```python
from build123d import *

# Parameters (mm, degrees)
F0_W     = 200
F0_H     = 172
F0_R     = 7.5
F1_DEPTH = 15
F2_T     = 2.5
F3_R     = 5


# Not quite as in the source:
# - a shell that OpenCascade refuses in one call is made with other operations: the cavity is built on its own and cut out


with BuildPart() as f1:
    # F0 (on Top) → F1 (new body)
    with BuildSketch(Plane.XY):
        with Locations((100, 86)):
            Rectangle(F0_W, F0_H)
        with Locations((11, 11)):
            Circle(F0_R, mode=Mode.SUBTRACT)
        with Locations((189, 11)):
            Circle(F0_R, mode=Mode.SUBTRACT)
        with Locations((11, 161)):
            Circle(F0_R, mode=Mode.SUBTRACT)
        with Locations((189, 161)):
            Circle(F0_R, mode=Mode.SUBTRACT)
    extrude(amount=F1_DEPTH)

    # F2: shell of thickness 2.5, made by hand


with BuildPart() as f2_core1:
    # F2_t2: copy of F1
    add(f1.part)

    # the walls: a layer under each face that stays
    f2_faces = [f2_core1.faces().sort_by_distance(p)[0] for p in [
        (0, 86, 7.5),
        (100, 0, 7.5),
        (200, 86, 7.5),
        (100, 172, 7.5),
        (3.5, 11, 7.5),
        (181.5, 11, 7.5),
        (3.5, 161, 7.5),
        (181.5, 161, 7.5),
        (100, 86, 0),
    ]]
    thicken(f2_faces, amount=-F2_T, mode=Mode.SUBTRACT)


with BuildPart() as f1_1:
    add(f1.part)

    # what is left inside the walls is the cavity
    f2_cavity = [f2_core1.part.solids().sort_by_distance(p)[0] for p in [
        (3.911255, 168.088745, 10.833333),
        (100, 58.166667, 14.975),
        (3.911255, 3.911255, 10.833333),
        (196.088745, 168.088745, 10.833333),
        (196.088745, 3.911255, 10.833333),
    ]]
    add(f2_cavity, mode=Mode.SUBTRACT)

    # F3
    f3_edges = [f1_1.edges().sort_by_distance(p)[0] for p in [
        (100, 169.5, 2.5),
        (16.267827, 169.5, 8.75),
        (183.732173, 169.5, 8.75),
        (18.071068, 153.928932, 2.5),
        (2.5, 155.732173, 8.75),
        (2.5, 86, 2.5),
        (2.5, 16.267827, 8.75),
        (18.071068, 18.071068, 2.5),
        (16.267827, 2.5, 8.75),
        (100, 2.5, 2.5),
        (183.732173, 2.5, 8.75),
        (181.928932, 18.071068, 2.5),
        (197.5, 16.267827, 8.75),
        (197.5, 86, 2.5),
        (197.5, 155.732173, 8.75),
        (181.928932, 153.928932, 2.5),
    ]]
    fillet(f3_edges, radius=F3_R)


solid = f1_1.part
```
Check sheet for the modelled part. Datum: model origin and axes. Units: mm. A direction names the side the tool comes from. Give positions to 0.01 mm unless a question says otherwise; leave off trailing zeros. Write each loop counter-clockwise with the first axis right and the second up, starting at its lowest first coordinate (ties: lowest second). Pieces come first, ordered by that corner, then holes.
Item 1: Draft check along Y on faces 3 (the face through (99, 0, 7)), 4 (the face through (21.699, 167.645, 11.198)), 5 (the face through (99, 87, 0)), 6 (the face through (195.546, 21.621, 11.198)). Enter one of: released by +Y, released by -Y, zero draft, split by the parting line, or undercut.
Item 2: Cross-section at D-D (y = 128). Enter the section's corners in (x, z).
Item 3: Gauge pin test, flat end, axial feed: pin 1 (4 mm diameter, centred on x = 52, y = 105.5, fed in from +Z). Record the tip position at first contact, or that the pin passes through.
Item 4: Access from +Z, -Z, +X, -X, +Y, -Y to the whole of each face (thin tool, end or side, straight path). Record for faces 1 (the face through (182.03, 18.17, 11.2)), 2 (the face through (195.93, 8.13, 7.4)).
Item 5: Cross-section at A-A (x = 189). Enter the section's corners in (y, z), and give its area (3 significant figures).
Item 6: Cross-section at C-C (x = 119). Enter the section's corners in (y, z), and give its area (3 significant figures).
Item 7: Cross-section at B-B (y = 11). Enter the section's corners in (x, z), and give its area (3 significant figures).
Item 8: Scan lines: L1, parallel to Y at x = 189, z = 8; L2, parallel to Y at x = 115.5, z = 7.5; L3, parallel to X at y = 31.5, z = 13.25. Record each from-to range of solid material in increasing order.
Report:
1. face 3: released by -Y
1. face 4: undercut
1. face 5: zero draft
1. face 6: undercut
2. outline: (0, 0) - (200, 0) - (200, 15) - (197.5, 15) - (197.5, 7.5) arc R5 cw to (192.5, 2.5) - (7.5, 2.5) arc R5 cw to (2.5, 7.5) - (2.5, 15) - (0, 15) - close
3. pin 1: stops at z = 2.5
4. face 1: +Z
4. face 2: +Z, -Z
5. outline: (0, 0) - (3.5, 0) - (3.5, 15) - (0, 15) - close; (18.5, 0) - (153.5, 0) - (153.5, 15) - (151, 15) - (151, 7.5) arc R5 cw to (146, 2.5) - (26, 2.5) arc R5 cw to (21, 7.5) - (21, 15) - (18.5, 15) - close; (168.5, 0) - (172, 0) - (172, 15) - (168.5, 15) - close
5. area: 516 mm2
6. outline: (0, 0) - (172, 0) - (172, 15) - (169.5, 15) - (169.5, 7.5) arc R5 cw to (164.5, 2.5) - (7.5, 2.5) arc R5 cw to (2.5, 7.5) - (2.5, 15) - (0, 15) - close
6. area: 503 mm2
7. outline: (0, 0) - (3.5, 0) - (3.5, 15) - (0, 15) - close; (18.5, 0) - (181.5, 0) - (181.5, 15) - (179, 15) - (179, 7.5) arc R5 cw to (174, 2.5) - (26, 2.5) arc R5 cw to (21, 7.5) - (21, 15) - (18.5, 15) - close; (196.5, 0) - (200, 0) - (200, 15) - (196.5, 15) - close
7. area: 586 mm2
8. L1: y = 0 to 3.5, 18.5 to 21, 151 to 153.5, 168.5 to 172
8. L2: y = 0 to 2.5, 169.5 to 172
8. L3: x = 0 to 2.5, 197.5 to 200
